Read the model definition and answer for the solid it produces. Units are mm, in the model's axes. Round coordinates to 2 decimals unless told otherwise and drop trailing zeros. Order: outer loops, then holes, each group sorted by start corner. A loop starts at its lowest first (then second) coordinate and runs counter-clockwise, first axis right, second up. Notation, with made-up numbers: M 62,-19.5 L 108,-19.5 A30 ccw 108,17.5 Z; hole C 9,3.25 d6. An arc over 180 degrees is marked long. Use one line per item in the form item = value. Start each with the question number.
from build123d import *

# Parameters (mm, degrees)
SKETCH_1_W      = 128.9
SKETCH_1_H      = 371.87
SKETCH_1_W_2    = 8
SKETCH_1_H_2    = 20
SKETCH_1_W_3    = 4
EXTRUDE_1_DEPTH = 4


with BuildPart() as part:
    # Эскиз1 → Бобышка-Вытянуть1 (new body)
    with BuildSketch(Plane(origin=(0, 0, 0), x_dir=(1, 0, 0), z_dir=(0, 1, 0))):
        with Locations((1.55, -185.935)):
            Rectangle(SKETCH_1_W, SKETCH_1_H)
        with Locations((0, -70)):
            Rectangle(SKETCH_1_W_2, SKETCH_1_H_2, mode=Mode.SUBTRACT)
        with Locations((0, -30)):
            Rectangle(SKETCH_1_W_2, SKETCH_1_H_2, mode=Mode.SUBTRACT)
        with Locations((0, -110)):
            Rectangle(SKETCH_1_W_2, SKETCH_1_H_2, mode=Mode.SUBTRACT)
        with Locations((0, -150)):
            Rectangle(SKETCH_1_W_2, SKETCH_1_H_2, mode=Mode.SUBTRACT)
        with Locations((0, -190)):
            Rectangle(SKETCH_1_W_2, SKETCH_1_H_2, mode=Mode.SUBTRACT)
        with Locations((0, -230)):
            Rectangle(SKETCH_1_W_2, SKETCH_1_H_2, mode=Mode.SUBTRACT)
        with Locations((0, -270)):
            Rectangle(SKETCH_1_W_2, SKETCH_1_H_2, mode=Mode.SUBTRACT)
        with Locations((0, -310)):
            Rectangle(SKETCH_1_W_2, SKETCH_1_H_2, mode=Mode.SUBTRACT)
        with Locations((0, -350)):
            Rectangle(SKETCH_1_W_2, SKETCH_1_H_2, mode=Mode.SUBTRACT)
        with Locations((-56.9, -30)):
            Rectangle(SKETCH_1_W_3, SKETCH_1_H_2, mode=Mode.SUBTRACT)
        with Locations((-56.9, -70)):
            Rectangle(SKETCH_1_W_3, SKETCH_1_H_2, mode=Mode.SUBTRACT)
        with Locations((-56.9, -110)):
            Rectangle(SKETCH_1_W_3, SKETCH_1_H_2, mode=Mode.SUBTRACT)
        with Locations((-56.9, -150)):
            Rectangle(SKETCH_1_W_3, SKETCH_1_H_2, mode=Mode.SUBTRACT)
        with Locations((-56.9, -190)):
            Rectangle(SKETCH_1_W_3, SKETCH_1_H_2, mode=Mode.SUBTRACT)
        with Locations((-56.9, -230)):
            Rectangle(SKETCH_1_W_3, SKETCH_1_H_2, mode=Mode.SUBTRACT)
        with Locations((-56.9, -270)):
            Rectangle(SKETCH_1_W_3, SKETCH_1_H_2, mode=Mode.SUBTRACT)
        with Locations((-56.9, -310)):
            Rectangle(SKETCH_1_W_3, SKETCH_1_H_2, mode=Mode.SUBTRACT)
        with Locations((-56.9, -350)):
            Rectangle(SKETCH_1_W_3, SKETCH_1_H_2, mode=Mode.SUBTRACT)
        with Locations((60, -70)):
            Rectangle(SKETCH_1_W_3, SKETCH_1_H_2, mode=Mode.SUBTRACT)
        with Locations((60, -30)):
            Rectangle(SKETCH_1_W_3, SKETCH_1_H_2, mode=Mode.SUBTRACT)
        with Locations((60, -110)):
            Rectangle(SKETCH_1_W_3, SKETCH_1_H_2, mode=Mode.SUBTRACT)
        with Locations((60, -150)):
            Rectangle(SKETCH_1_W_3, SKETCH_1_H_2, mode=Mode.SUBTRACT)
        with Locations((60, -190)):
            Rectangle(SKETCH_1_W_3, SKETCH_1_H_2, mode=Mode.SUBTRACT)
        with Locations((60, -230)):
            Rectangle(SKETCH_1_W_3, SKETCH_1_H_2, mode=Mode.SUBTRACT)
        with Locations((60, -270)):
            Rectangle(SKETCH_1_W_3, SKETCH_1_H_2, mode=Mode.SUBTRACT)
        with Locations((60, -310)):
            Rectangle(SKETCH_1_W_3, SKETCH_1_H_2, mode=Mode.SUBTRACT)
        with Locations((60, -350)):
            Rectangle(SKETCH_1_W_3, SKETCH_1_H_2, mode=Mode.SUBTRACT)
    extrude(amount=EXTRUDE_1_DEPTH)


solid = part.part
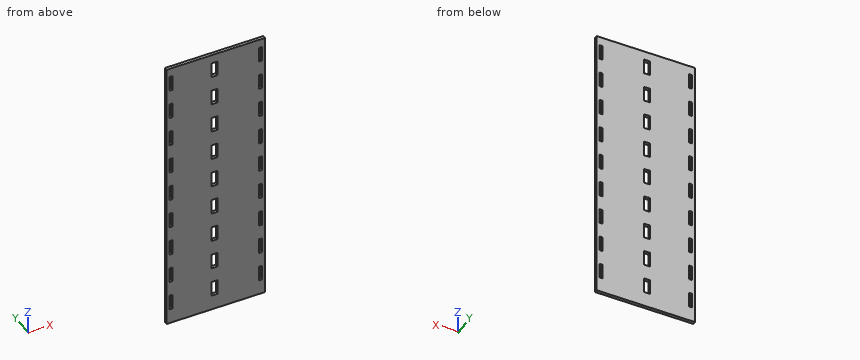
Item 1: Section A-A (z = 304) is taken. Write down the section's boundary in (x, y), and give its area (3 significant figures).
Item 2: Section B-B (y = 2.1) is taken. Give the number of separate pieces and of enclosed holes in the cut face, and give its area (3 significant figures).
Item 3: Find the intervals of material crossed by L1, parallel to X at y = 2.55, z = 275, in increasing order. Write a range as [from, to].
The answers:
q1.outline = M -62.9,0 L -58.9,0 L -58.9,4 L -62.9,4 Z; M -54.9,0 L -4,0 L -4,4 L -54.9,4 Z; M 4,0 L 58,0 L 58,4 L 4,4 Z; M 62,0 L 66,0 L 66,4 L 62,4 Z
q1.area = 452 mm²
q2.separate_pieces = 1
q2.enclosed_holes = 27
q2.area = 45,100 mm²
q3.L1 = [-62.9, -58.9], [-54.9, -4], [4, 58], [62, 66]
